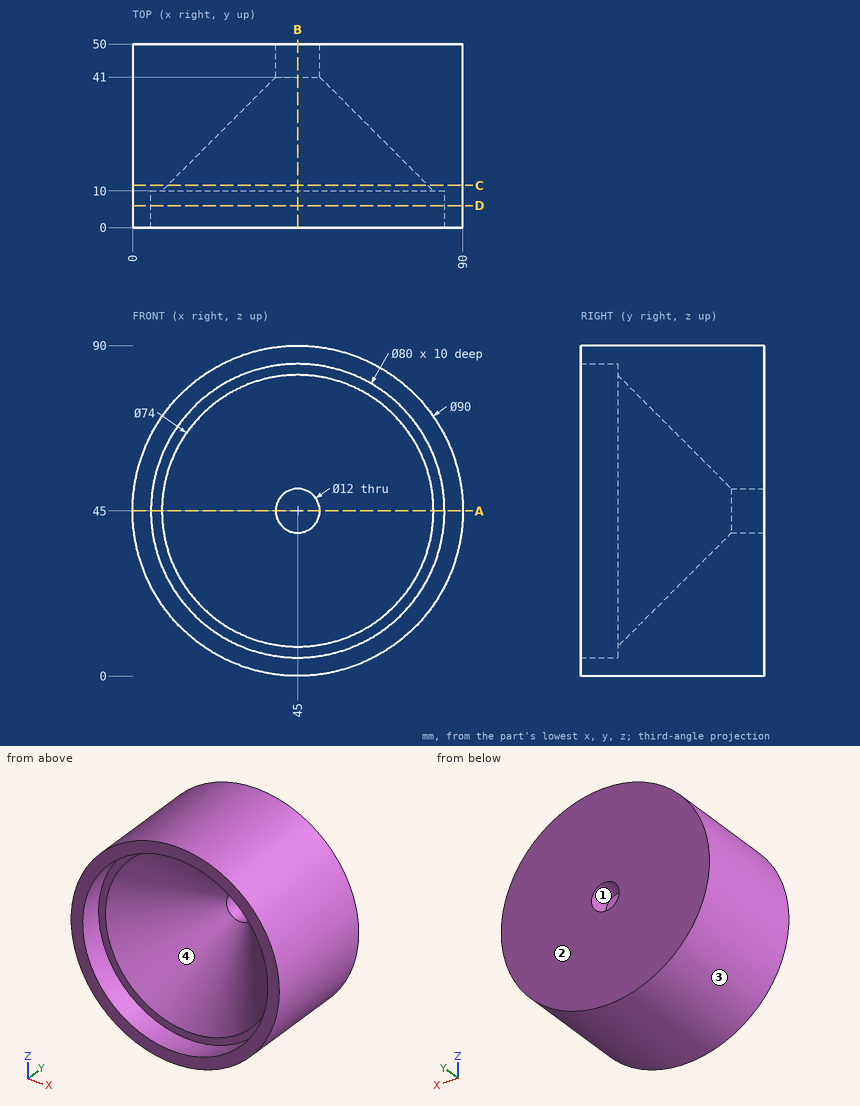
Verification items for this drawing (mm, ordinates from the low corner). Give positions to 0.01 mm unless a question says otherwise; leave off trailing zeros. Write each loop counter-clockwise with the first axis right and the second up, starting at its lowest first coordinate (ties: lowest second). Pieces come first, ordered by that corner, then holes. Notation, with made-up numbers: (-9, -22) - (17, -22) arc R18 ccw to (17, -10) - close; hole circle Ø10 at (60, -11.5). An arc over 180 degrees is marked (long way). Answer as CSV lines item,"result". Start each with the question number.
1. Sectioned sample at D-D (y = 6). Record the boundary of the cut face in (x, z), then the cut area to 3 significant figures.
2. Depth check by flat-ended pin: pin 1 (1.5 mm diameter, centred on y = 8, z = 25.5, fed in from +X); pin 2 (11 mm diameter, centred on x = 45, z = 45, fed in from +Y); pin 3 (1 mm diameter, centred on x = 35.5, z = 59.5, fed in from -Y); pin 4 (12 mm diameter, centred on x = 18.5, y = 41.5, fed in from +Z). Enter the tip coordinate at first touch or a pass-through.
3. Draft check along X on the marked faces 1, 2, 3 and 4. Enter one of: pulls with the +X half, pulls with the -X half, needs draft (parallel to the pull), parting line crosses it, or undercut.
4. Sectioned sample at A-A (z = 45). Record the boundary of the cut face in (x, y).
5. Sectioned sample at B-B (x = 45). Record the boundary of the cut face in (y, z).
6. Sectioned sample at C-C (y = 11.5). Record the boundary of the cut face in (x, z), then the cut area to 3 significant figures.
7. Thickness scan on line 1 (Z direction, x = 45, y = 46.5); line 2 (Z direction, x = 45, y = 5.25). Record the ranges inside material, lowest first.
Derived:
1,outline,"circle Ø90 at (45, 45); hole circle Ø80 at (45, 45)"
1,area,"1,340 mm²"
2,pin 1,"x = 85.91"
2,pin 2,"through"
2,pin 3,"y = 29.17"
2,pin 4,"z = 85.06"
3,face 1,"undercut"
3,face 2,"needs draft"
3,face 3,"parting line crosses it"
3,face 4,"undercut"
4,outline,"(0, 0) - (5, 0) - (5, 10) - (8, 10) - (39, 41) - (39, 50) - (0, 50) - close; (51, 41) - (82, 10) - (85, 10) - (85, 0) - (90, 0) - (90, 50) - (51, 50) - close"
5,outline,"(0, 0) - (50, 0) - (50, 39) - (41, 39) - (10, 8) - (10, 5) - (0, 5) - close; (0, 85) - (10, 85) - (10, 82) - (41, 51) - (50, 51) - (50, 90) - (0, 90) - close"
6,outline,"circle Ø90 at (45, 45); hole circle Ø71 at (45, 45)"
6,area,"2,400 mm²"
7,line 1,"0 to 39, 51 to 90"
7,line 2,"0 to 5, 85 to 90"
